from build123d import *

# Parameters (mm, degrees)
EXTRUDE_THIN1_DEPTH = 206.375
FILLET1_R           = 1.27


with BuildPart() as part:
    # Sketch1 → Extrude-Thin1 (new body)
    with BuildSketch(Plane.XY):
        with BuildLine():
            Line((0, 7.9375), (0, 3.96875))
            ThreePointArc((0, 3.96875), (-3.354205948, 3.225220302), (-6.080014609, 1.133928571))
            ThreePointArc((-6.080014609, 1.133928571), (-9.057226525, 0.047161235), (-11.491167025, 2.077133569))
            Line((-11.491167025, 2.077133569), (-12.480770453, 4.7625))
            Line((-12.480770453, 4.7625), (-14.068270453, 4.7625))
            Line((-14.068270453, 4.7625), (-14.068270453, 8.407719714))
            ThreePointArc((-14.068270453, 8.407719714), (-15.883557794, 14.00110471), (-20.6375, 17.4625))
            Line((-20.6375, 17.4625), (-20.6375, 21.43125))
            Line((-20.6375, 21.43125), (-16.66875, 21.43125))
            Line((-16.66875, 21.43125), (-16.66875, 20.16125))
            Line((-16.66875, 20.16125), (-19.3675, 20.16125))
            Line((-19.3675, 20.16125), (-19.3675, 18.341243212))
            ThreePointArc((-19.3675, 18.341243212), (-14.589126489, 14.362332756), (-12.798270453, 8.407719714))
            Line((-12.798270453, 8.407719714), (-12.798270453, 6.0325))
            Line((-12.798270453, 6.0325), (-11.595295513, 6.0325))
            Line((-11.595295513, 6.0325), (-10.299508396, 2.516280141))
            ThreePointArc((-10.299508396, 2.516280141), (-8.839144096, 1.298296741), (-7.052816947, 1.950357143))
            ThreePointArc((-7.052816947, 1.950357143), (-4.458468146, 4.08731095), (-1.27, 5.150743201))
            Line((-1.27, 5.150743201), (-1.27, 7.9375))
            Line((-1.27, 7.9375), (0, 7.9375))
        make_face()
    extrude(amount=-EXTRUDE_THIN1_DEPTH)

    # Fillet1
    fillet1_edges = [part.edges().sort_by_distance(p)[0] for p in [
        (-11.595295513, 6.0325, -103.1875),
        (0, 3.96875, -103.1875),
        (-14.068270453, 4.7625, -103.1875),
        (-20.6375, 17.4625, -103.1875),
        (-20.6375, 21.43125, -103.1875),
    ]]
    fillet(fillet1_edges, radius=FILLET1_R)


solid = part.part
Could you check a few things on this model? Use its own coordinates, in mm. A direction names the side the tool comes from. Give positions to 0.01 mm unless a question says otherwise; leave off trailing zeros. Loops run counter-clockwise (first coordinate to the right, second up) from the corner with the lowest first, then second, coordinate; pieces in that order, holes last. Notation, with made-up numbers: (17, -10.5) -> (55, -10.5) arc R10 ccw to (55, -2.5) -> close; hole circle Ø6 at (39.5, -33). An arc over 180 degrees is marked (long way). Answer as CSV lines item,"result". Start each with the question number.
(1) If we section it at B-B on y = 12: Write out the boundary of the cut face in (x, z) (1 decimal), then the cut area to 3 significant figures.
(2) I'm going to push flat-ended pins straight in: pin 1 Ø5 at (y, z) = (15.5, -134) entering from -X; pin 2 Ø1.4 at (y, z) = (7, -79) entering from -X; pin 3 Ø1 at (y, z) = (10, -163.5) entering from +X. Where does each tip first touch, or does it pass through?
(3) We'd pull the mould along X, two halves only. Please class faces 3 (the cylindrical face through (-3.8, 3, -101.7)), 4 (the cylindrical face through (-4.5, 4.064, -101.743)), 5 (the flat face through (-13.3, 10, 0)): released by +X, released by -X, zero draft, split by the parting line, or undercut.
(4) I need wall thicknesses on probe 1 along Y at (x, z) = (-17.5, -143.5); probe 2 along X at (y, z) = (1.5, -27.5); probe 3 along X at (y, z) = (8.5, -164.5). Which ranges of each line are inside material? Lowest first, please.
(5) Which directions (+Z, -Z, +X, -X, +Y, -Y) give clear straight access to the entire face, cutting with the end or side of a thin tool? Please do faces 1 (the cylindrical face through (-14.64, 14.44, -101.74)), 2 (the cylindrical face through (-15.61, 13.6, -101.74)).
Computed:
1,outline,"(-14.8, -206.4) -> (-13.4, -206.4) -> (-13.4, 0) -> (-14.8, 0) -> close"
1,area,"280 mm2"
2,pin 1,"stops at x = -20.59"
2,pin 2,"stops at x = -14.07"
2,pin 3,"stops at x = -12.85"
3,face 3,"released by +X"
3,face 4,"undercut"
3,face 5,"zero draft"
4,probe 1,"y = 15.73 to 17.32, 20.16 to 21.43"
4,probe 2,"x = -11.21 to -9.42, -7.6 to -5.75"
4,probe 3,"x = -14.07 to -12.8"
5,face 1,"+Z, -Z, +X"
5,face 2,"+Z, -Z, -X, -Y"
